```python
from build123d import *

# Parameters (mm, degrees)
BASE_FLANGE1_DEPTH = 17.4625
SKETCH6_R          = 2.54
CUT_EXTRUDE1_DEPTH = 2.54
SKETCH7_R          = 2.54
CUT_EXTRUDE2_DEPTH = 2.54


# Sheet-metal steps are written as plain solids
with BuildPart() as part:
    # Sketch1 → Base-Flange1 (new, symmetric)
    with BuildSketch(Plane(origin=(0, 0, 0), x_dir=(0, 0, -1), z_dir=(1, 0, 0))):
        with BuildLine():
            Line((0, 0), (0, 23.8125))
            ThreePointArc((0, 23.8125), (0.464967985, 24.935032015), (1.5875, 25.4))
            Line((1.5875, 25.4), (50.8, 25.4))
            Line((50.8, 25.4), (50.8, 26.9875))
            Line((50.8, 26.9875), (1.5875, 26.9875))
            ThreePointArc((1.5875, 26.9875), (-0.65756403, 26.05756403), (-1.5875, 23.8125))
            Line((-1.5875, 23.8125), (-1.5875, 0))
            Line((-1.5875, 0), (0, 0))
        make_face()
    extrude(amount=BASE_FLANGE1_DEPTH, both=True)

    # Sketch6 → Cut-Extrude1 (cut)
    with BuildSketch(Plane.XY.offset(1.5875)):
        with Locations((-8.73125, 11.90625)):
            Circle(SKETCH6_R)
        with Locations((8.73125, 11.90625)):
            Circle(SKETCH6_R)
    extrude(amount=-CUT_EXTRUDE1_DEPTH, mode=Mode.SUBTRACT)

    # Sketch7 → Cut-Extrude2 (cut)
    with BuildSketch(Plane(origin=(0, 26.9875, 0), x_dir=(1, 0, 0), z_dir=(0, 1, 0))):
        with Locations(Location((-8.73125, 38.1, 0), (0, 0, 270))):
            Circle(SKETCH7_R)
        with Locations(Location((8.73125, 38.1, 0), (0, 0, 270))):
            Circle(SKETCH7_R)
    extrude(amount=-CUT_EXTRUDE2_DEPTH, mode=Mode.SUBTRACT)


solid = part.part
```
Here's how the part is built. I have some questions about the finished solid (model axes, mm). A direction names the side the tool comes from. Round coordinates to 2 decimals unless told otherwise and drop trailing zeros. Order: outer loops, then holes, each group sorted by start corner. A loop starts at its lowest first (then second) coordinate and runs counter-clockwise, first axis right, second up. Notation, with made-up numbers: (15.5, 80) -> (27.5, 80) arc R8 ccw to (27.5, 88) -> close; hole circle Ø7 at (75, 4.5). An arc over 180 degrees is marked (long way). Use a Markdown table: item, result. Add a question column.
(1) I need wall thicknesses on line 1 along X through (y, z) = (26.65, -38.1); line 2 along Z through (x, y) = (11, 14.75); line 3 along Y through (x, z) = (1.5, -9). Which ranges of each line are inside material? Lowest first, please.
(2) For faces 4 (the face through (0, 12, 0)), 5 (the face through (8.181, 9.427, 0.805)), which set-ups out of +Z, -Z, +X, -X, +Y, -Y let a thin tool reach every point of the face, with its end or its side?
(3) If we mould it in two halves opening along X, with no side actions, what happens to faces 1 (the face through (11.25, 26.2, -38.43)), 2 (the face through (-17.462, 26, -17)), 3 (the face through (0, 25.4, -26))? For each: released by +X, released by -X, zero draft, split by the parting line, or undercut.
(4) For pin 1 Ø2 at (x, z) = (1, -40) entering from -Y; pin 2 Ø4 at (x, z) = (-8.73, -38.1) entering from -Y; pin 3 Ø5 at (x, y) = (3, 11.5) entering from -Z, each with a flat end and sliding along its axis, tell me the tip position at first contact or that it passes through.
(5) Suppose I cut it at C-C, the plane y = 22. Please give me the cut outline in (x, z).
(6) Suppose I cut it at D-D, the plane z = -9. Please give me the cut outline in (x, y).
(7) Suppose I cut it at A-A, the plane z = -38.1. Please give me the cut outline in (x, y), and give its area (3 significant figures).
Verdict:
| question | item | result |
|---|---|---|
| 1 | line 1 | -17.46 to -11.27, -6.19 to 6.19, 11.27 to 17.46 |
| 1 | line 2 | 0 to 1.59 |
| 1 | line 3 | 25.4 to 26.99 |
| 2 | face 4 | -Z, +X, -X, -Y |
| 2 | face 5 | +Z, -Z |
| 3 | face 1 | undercut |
| 3 | face 2 | released by -X |
| 3 | face 3 | zero draft |
| 4 | pin 1 | y = 25.4 |
| 4 | pin 2 | through |
| 4 | pin 3 | z = 0 |
| 5 | outline | (-17.46, 0) -> (17.46, 0) -> (17.46, 1.59) -> (-17.46, 1.59) -> close |
| 6 | outline | (-17.46, 25.4) -> (17.46, 25.4) -> (17.46, 26.99) -> (-17.46, 26.99) -> close |
| 7 | outline | (-17.46, 25.4) -> (-11.27, 25.4) -> (-11.27, 26.99) -> (-17.46, 26.99) -> close; (-6.19, 25.4) -> (6.19, 25.4) -> (6.19, 26.99) -> (-6.19, 26.99) -> close; (11.27, 25.4) -> (17.46, 25.4) -> (17.46, 26.99) -> (11.27, 26.99) -> close |
| 7 | area | 39.3 mm2 |
